```python
from build123d import *

# Parameters (mm, degrees)
F1_DEPTH = 152.4
F2_R     = 1.98374
F3_R     = 3.69316
F4_R     = 3.175
F5_R     = 9.525
F5_R_2   = 1.8288
F6_DEPTH = 155.81884
F7_R     = 60.500006
F8_DEPTH = 1.70942


with BuildPart() as f1:
    # F0 (on Top) → F1 (new body)
    with BuildSketch(Plane.XY):
        Polygon((0, 32.3337428), (0, 0), (-152.4, 0), (-152.4, 32.3337428), (-154.10942, 32.3337428), (-154.10942, -1.70942), (1.70942, -1.70942), (1.70942, 32.3337428), align=None)
    extrude(amount=F1_DEPTH)

    # F2
    f2_edges = [f1.edges().sort_by_distance(p)[0] for p in [
        (0, 0, 76.2),
        (-152.4, 0, 76.2),
    ]]
    fillet(f2_edges, radius=F2_R)

    # F3
    f3_edges = [f1.edges().sort_by_distance(p)[0] for p in [
        (1.70942, -1.70942, 76.2),
        (-154.10942, -1.70942, 76.2),
    ]]
    fillet(f3_edges, radius=F3_R)

    # F4
    f4_edges = [f1.edges().sort_by_distance(p)[0] for p in [
        (-153.25471, 32.333743, 0),
        (0.85471, 32.333743, 0),
    ]]
    fillet(f4_edges, radius=F4_R)

    # F5 (on face) → F6 (cut, through all)
    with BuildSketch(Plane.YZ.offset(1.70942)):
        with Locations((19.0559546638, 13.2777881362)):
            Circle(F5_R)
        with Locations((29.1587428, 23.3805762724)):
            Circle(F5_R_2)
        with Locations((29.1587428, 3.175)):
            Circle(F5_R_2)
        with Locations((8.9531665276, 3.175)):
            Circle(F5_R_2)
        with Locations((8.9531665276, 23.3805762724)):
            Circle(F5_R_2)
    extrude(amount=-F6_DEPTH, mode=Mode.SUBTRACT)

    # F7 (on face) → F8 (cut, through all)
    with BuildSketch(Plane.XZ.offset(1.70942)):
        with Locations((-76.2, 76.2)):
            Circle(F7_R)
    extrude(amount=-F8_DEPTH, mode=Mode.SUBTRACT)


solid = f1.part
```
Geometry: final body of the model. Coordinates: model frame, mm. A direction names the side the tool comes from. Coordinates: 2 decimals unless noted, no trailing zeros. Write each loop counter-clockwise with the first axis right and the second up, starting at its lowest first coordinate (ties: lowest second). Pieces come first, ordered by that corner, then holes. Notation, with made-up numbers: M -15,34.25 L 38,34.25 A25 cw 38,69.25 Z; hole C 55,37.5 d10. An arc over 180 degrees is marked long. Answer as CSV lines item,"result". Start each with the question number.
Q1. Mould query, pull axis Y, two halves, no side actions, for faces 3 (the cylindrical face through (0.867, 7.126, 3.255)), 4 (the flat face through (0, 17, 75)), 5 (the cylindrical face through (0.656, -0.599, 77.267)), 6 (the cylindrical face through (0.867, 28.762, 21.595)). Classes: released by +Y, released by -Y, zero draft, split by the parting line, or undercut.
Q2. Cut plane C-C on y = 23. Return the cut outline in (x, z), then the cut area to 3 significant figures.
Q3. Cut plane B-B on z = 76.2. Return the cut outline in (x, y), then the cut area to 3 significant figures.
Q4. Line query: line 1 (X direction, y = 14, z = 42.5); line 2 (Y direction, x = -141, z = 135). Output: solid intervals per line, ascending. Write a range as from..to.
Q5. Cut plane A-A on x = -76.2. Return the cut outline in (y, z).
Q6. Pin query (flat end, axial travel): P1, Ø4, axis at y = 29.16, z = 3.18, coming from the +X side; P2, Ø1.5, axis at x = -15, z = 115.5, coming from the +Y side. Return the tip coordinate at first contact, or that it passes through.
Q7. Reachability of faces 1 (the cylindrical face through (-153.243, 28.762, 21.595)), 2 (the flat face through (-42, 0, 24)) from +Z, -Z, +X, -X, +Y, -Y: full face, straight path, thin tool, end or side. Return the list, or none.
Q8. Cut plane D-D on x = -44.5. Return the cut outline in (y, z).
Findings below:
1,face 3,"undercut"
1,face 4,"zero draft"
1,face 5,"released by -Y"
1,face 6,"undercut"
2,outline,"M -154.11,0 L -152.4,0 L -152.4,4.61 L -154.11,4.61 Z; M -154.11,21.95 L -152.4,21.95 L -152.4,152.4 L -154.11,152.4 Z; M 0,0 L 1.71,0 L 1.71,4.61 L 0,4.61 Z; M 0,21.95 L 1.71,21.95 L 1.71,152.4 L 0,152.4 Z"
2,area,"462 mm2"
3,outline,"M -154.11,1.98 A3.69 ccw -150.42,-1.71 L -136.7,-1.71 L -136.7,0 L -150.42,0 A1.98 cw -152.4,1.98 L -152.4,32.33 L -154.11,32.33 Z; M -15.7,-1.71 L -1.98,-1.71 A3.69 ccw 1.71,1.98 L 1.71,32.33 L 0,32.33 L 0,1.98 A1.98 cw -1.98,0 L -15.7,0 Z"
3,area,"166 mm2"
4,line 1,"x = -154.11..-152.4, 0..1.71"
4,line 2,"y = -1.71..0"
5,outline,"M -1.71,0 L 0,0 L 0,15.7 L -1.71,15.7 Z; M -1.71,136.7 L 0,136.7 L 0,152.4 L -1.71,152.4 Z"
6,P1,"stops at x = 1.71"
6,P2,"stops at y = 0"
7,face 1,"+X, -X"
7,face 2,"+Z, -Z, +Y"
8,outline,"M -1.71,0 L 0,0 L 0,24.67 L -1.71,24.67 Z; M -1.71,127.73 L 0,127.73 L 0,152.4 L -1.71,152.4 Z"
